The listing builds one solid part. Answer for the finished solid, in the listing's coordinates (mm). Face numbers are marked on the shaded views. A direction names the side the tool comes from. Give positions to 0.01 mm unless a question says otherwise; leave off trailing zeros. Order: outer loops, then holes, each group sorted by start corner. A loop starts at its lowest first (then second) coordinate and runs counter-clockwise, first axis right, second up. Notation, with made-up numbers: (85.25, 6) -> (130.25, 6) arc R16 ccw to (130.25, 27) -> close; hole circle Ø3 at (56, 45). An arc over 180 degrees is marked (long way). Answer as a JSON object with one key per item and string values. Group by question number.
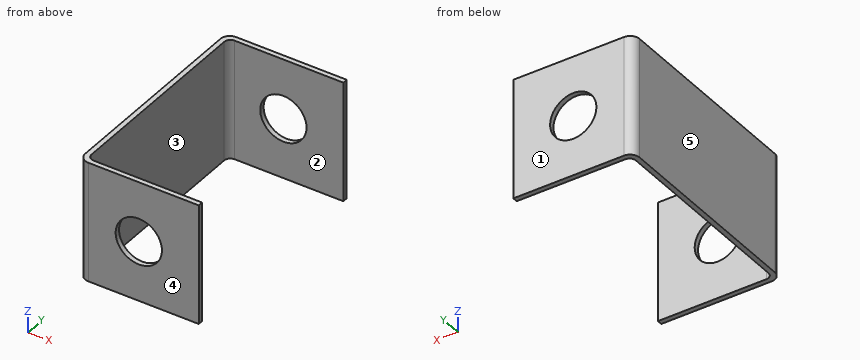
```python
from build123d import *

# Parameters (mm, degrees)
BOSS_EXTRUDE1_DEPTH = 38.1
SKETCH3_R           = 7.35
CUT_EXTRUDE1_DEPTH  = 82.664668768
FILLET1_R           = 2
FILLET2_R           = 3


with BuildPart() as part:
    # Sketch1 → Boss-Extrude1 (new body)
    with BuildSketch(Plane.XY):
        Polygon((-17.4625, 68.0875), (19.05, 68.0875), (19.05, 69.675), (-19.05, 69.675), (-19.05, 0), (19.05, 0), (19.05, 1.5875), (-17.4625, 1.5875), align=None)
    extrude(amount=BOSS_EXTRUDE1_DEPTH)

    # Sketch3 → Cut-Extrude1 (cut, through all)
    with BuildSketch(Plane(origin=(0, 0, 0), x_dir=(1, 0, 0), z_dir=(0, 1, 0))):
        with Locations((0, -19.05)):
            Circle(SKETCH3_R)
    extrude(amount=CUT_EXTRUDE1_DEPTH, mode=Mode.SUBTRACT)

    # Fillet1
    fillet1_edges = [part.edges().sort_by_distance(p)[0] for p in [
        (-17.4625, 1.5875, 19.05),
        (-17.4625, 68.0875, 19.05),
    ]]
    fillet(fillet1_edges, radius=FILLET1_R)

    # Fillet2
    fillet2_edges = [part.edges().sort_by_distance(p)[0] for p in [
        (-19.05, 0, 19.05),
        (-19.05, 69.675, 19.05),
    ]]
    fillet(fillet2_edges, radius=FILLET2_R)


solid = part.part
```
(1) A cutting plane is placed at B-B (x = -9). Determine the outline of the cut face in (y, z) (1 decimal).
(2) Flat-ended cylindrical pins translate along their axes: pin 1 Ø2 at (y, z) = (21.5, 13.5) entering from +X; pin 2 Ø9 at (x, z) = (0, 19.05) entering from -Y. Find the tip coordinate at first contact, or state that the pin passes through.
(3) A cutting plane is placed at C-C (x = 0). Determine the outline of the cut face in (y, z) (1 decimal).
(4) For a pull along Y with two mould halves and no side action, classify the marked faces 3, 4 and 5 as +Y half, -Y half, draft (parallel to the pull), parting line (faces both ways), or undercut.
(5) A cutting plane is placed at A-A (z = 19.05). State how many separate pieces and enclosed holes the cut face has, and give its area (3 significant figures).
(6) Find the intervals of material crossed by line 1 along Y through (x, z) = (-8.5, 34.5) (1 decimal); line 2 along Z through (x, y) = (0, 69.3); line 3 along X through (y, z) = (30.5, 32), in increasing order. Write a range as [from, to].
(7) Which of the six approach directions +Z, -Z, +X, -X, +Y, -Y give full straight-line access (tool end or side, diameter ignored) to the marked faces 1 and 2?
Check sheet entries:
{
 "1": {"outline": "(0, 0) -> (1.6, 0) -> (1.6, 38.1) -> (0, 38.1) -> close; (68.1, 0) -> (69.7, 0) -> (69.7, 38.1) -> (68.1, 38.1) -> close"},
 "2": {"pin 1": "stops at x = -17.46", "pin 2": "passes through"},
 "3": {"outline": "(0, 0) -> (1.6, 0) -> (1.6, 11.7) -> (0, 11.7) -> close; (0, 26.4) -> (1.6, 26.4) -> (1.6, 38.1) -> (0, 38.1) -> close; (68.1, 0) -> (69.7, 0) -> (69.7, 11.7) -> (68.1, 11.7) -> close; (68.1, 26.4) -> (69.7, 26.4) -> (69.7, 38.1) -> (68.1, 38.1) -> close"},
 "4": {"face 3": "undercut", "face 4": "-Y half", "face 5": "draft"},
 "5": {"separate pieces": "3", "enclosed holes": "0", "area": "178 mm2"},
 "6": {"line 1": "y = [0, 1.6], [68.1, 69.7]", "line 2": "z = [0, 11.7], [26.4, 38.1]", "line 3": "x = [-19.05, -17.46]"},
 "7": {"face 1": "+Z, -Z, +X, -X, +Y", "face 2": "+Z, -Z, +X"}
}
